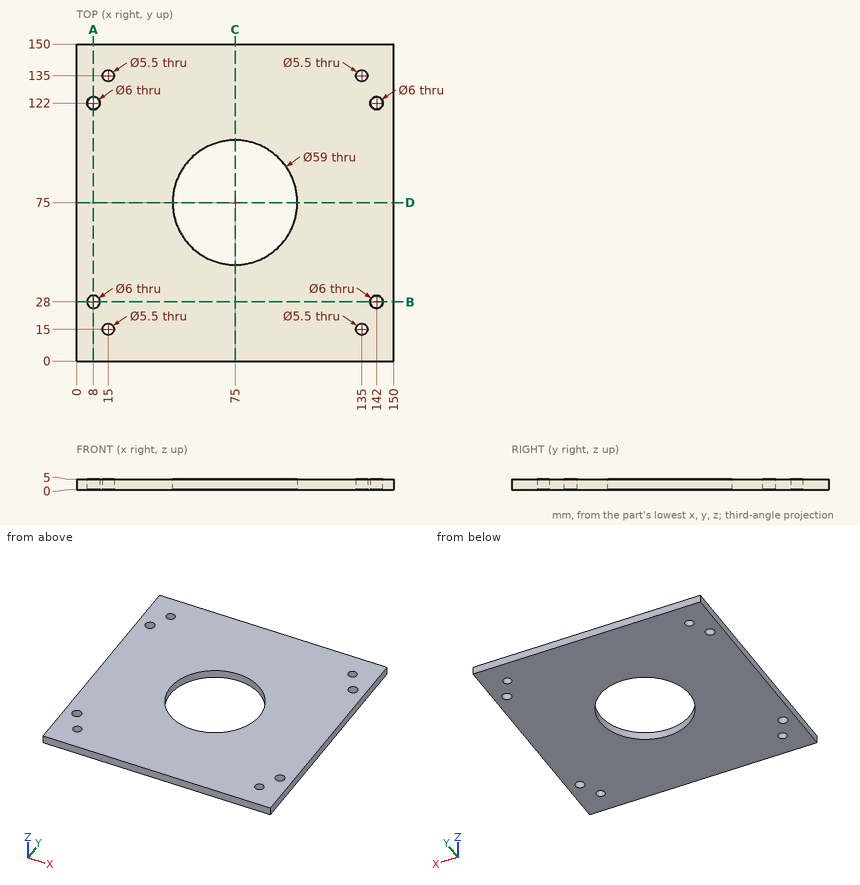
Design review of the part shown in the three views and the two pictorial views. Dimensions are in mm from the part's minimum x, y and z. Give positions to 0.01 mm unless a question says otherwise; leave off trailing zeros. Loops run counter-clockwise (first coordinate to the right, second up) from the corner with the lowest first, then second, coordinate; pieces in that order, holes last. Notation, with made-up numbers: (9, 86.5) -> (59, 86.5) arc R29 ccw to (59, 108.5) -> close; hole circle Ø9 at (-3.75, 32.25). An arc over 180 degrees is marked (long way). One line per item, written item: value.
Q1. We need section C-C on x = 75. Give the boundary of the cut face in (y, z), and give its area (3 significant figures).
Numbers:
outline: (0, 0) -> (45.5, 0) -> (45.5, 5) -> (0, 5) -> close; (104.5, 0) -> (150, 0) -> (150, 5) -> (104.5, 5) -> close
area: 455 mm^2
Q2. We need section B-B on y = 28. Give the boundary of the cut face in (x, z), and give its area (3 significant figures).
Numbers:
outline: (0, 0) -> (5, 0) -> (5, 5) -> (0, 5) -> close; (11, 0) -> (139, 0) -> (139, 5) -> (11, 5) -> close; (145, 0) -> (150, 0) -> (150, 5) -> (145, 5) -> close
area: 690 mm^2
Q3. For L1, parallel to Y at x = 8, z = 2.1; L2, parallel to X at y = 135, z = 3.75; L3, parallel to X at y = 122, z = 1.45, list the stretches that pass through material, from the lowest coordinate up.
Numbers:
L1: y = 0 to 25, 31 to 119, 125 to 150
L2: x = 0 to 12.25, 17.75 to 132.25, 137.75 to 150
L3: x = 0 to 5, 11 to 139, 145 to 150
Q4. We need section A-A on x = 8. Give the boundary of the cut face in (y, z).
Numbers:
outline: (0, 0) -> (25, 0) -> (25, 5) -> (0, 5) -> close; (31, 0) -> (119, 0) -> (119, 5) -> (31, 5) -> close; (125, 0) -> (150, 0) -> (150, 5) -> (125, 5) -> close
